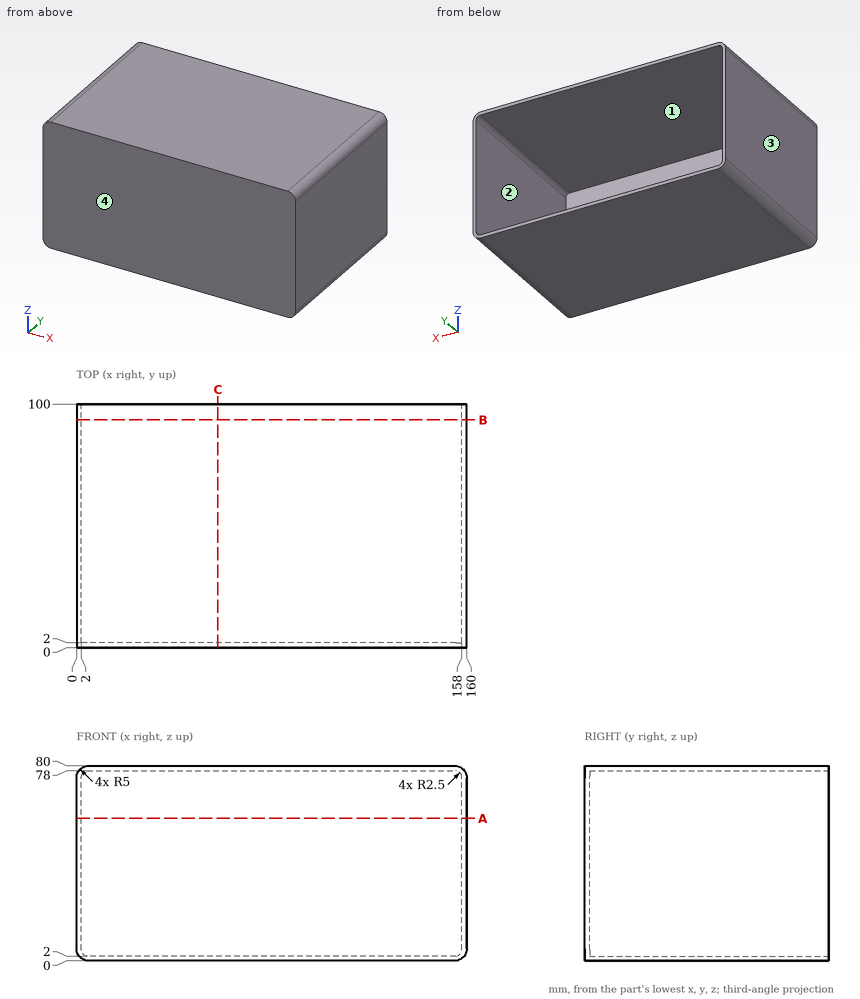
Design review of the part shown in the three views and the two pictorial views. Dimensions are in mm from the part's minimum x, y and z. Coordinates: 2 decimals unless noted, no trailing zeros. Loops run counter-clockwise (first coordinate to the right, second up) from the corner with the lowest first, then second, coordinate; pieces in that order, holes last.
(1) Consider section A-A, the plane z = 58.5. Give the boundary of the cut face in (x, y), plus the area to 3 significant figures.
Determined:
outline: (0, 0) - (160, 0) - (160, 100) - (158, 100) - (158, 2) - (2, 2) - (2, 100) - (0, 100) - close
area: 712 mm2
(2) Draft analysis for pull direction X (two halves, no side actions). For the marked faces 1, 2, 3 and 4, state which applies: +X half, -X half, draft (parallel to the pull), parting line (faces both ways), or undercut.
Determined:
face 1: undercut
face 2: undercut
face 3: -X half
face 4: draft
(3) Wall thickness on L1, parallel to X at y = 40.5, z = 43.5; L2, parallel to Z at x = 71.5, y = 38; L3, parallel to Y at x = 139.5, z = 21: over which ranges is each line inside the solid? List them lowest first.
Determined:
L1: x = 0 to 2, 158 to 160
L2: z = 0 to 2, 78 to 80
L3: y = 0 to 2
(4) Consider section C-C, the plane x = 58. Give the boundary of the cut face in (y, z).
Determined:
outline: (0, 0) - (100, 0) - (100, 2) - (2, 2) - (2, 78) - (100, 78) - (100, 80) - (0, 80) - close
(5) Insertion check: P1, Ø6, axis at y = 65, z = 27.5, coming from the -X side; P2, Ø1.5, axis at x = 22, z = 46, coming from the +Y side. Each pin has a flat end and moves straight along its axis. Give the tip position at first contact, or say it passes through.
Determined:
P1: stops at x = 0
P2: stops at y = 2
(6) Consider section B-B, the plane y = 93.5. Give the boundary of the cut face in (x, z), plus the area to 3 significant figures.
Determined:
outline: (0, 5) arc R5 ccw to (5, 0) - (155, 0) arc R5 ccw to (160, 5) - (160, 75) arc R5 ccw to (155, 80) - (5, 80) arc R5 ccw to (0, 75) - close; hole (2, 4.5) arc R2.5 ccw to (4.5, 2) - (155.5, 2) arc R2.5 ccw to (158, 4.5) - (158, 75.5) arc R2.5 ccw to (155.5, 78) - (4.5, 78) arc R2.5 ccw to (2, 75.5) - close
area: 928 mm2
